Here's how the part is built. I have some questions about the finished solid (model axes, mm). Face numbers are marked on the shaded views. Round coordinates to 2 decimals unless told otherwise and drop trailing zeros. Write each loop counter-clockwise with the first axis right and the second up, starting at its lowest first coordinate (ties: lowest second). Pieces come first, ordered by that corner, then holes. Notation, with made-up numbers: (44.25, -2) - (99.25, -2) arc R22 ccw to (99.25, 35) - close; hole circle Ø8 at (67, 36). An arc over 180 degrees is marked (long way). One line per item, written item: value. Start each with the question number.
Item 1: For P1, Ø2, axis at x = 41.5, z = 2.5, coming from the -Y side; P2, Ø1, axis at x = 45, z = 2, coming from the -Y side, each with a flat end and sliding along its axis, tell me the tip position at first contact or that it passes through.
Item 2: Imagine slicing it at D-D, the plane y = -24. Please give me the cut outline in (x, z), then the cut area to 3 significant figures.
Item 3: Imagine slicing it at A-A, the plane x = 46.25. Please give me the cut outline in (y, z).
Item 4: If I drill on line 1 (X direction, y = -28, z = 0.5); line 2 (X direction, y = -22.5, z = 2.85); line 3 (X direction, y = -29.75, z = 4.3), over which ranges is the centre line in solid material (lowest first)?
Item 5: Thinking about a two-plate mould opening in X: for the marked faces 1, 2 and 3, which applies, released by +X, released by -X, zero draft, split by the parting line, or undercut?
Item 6: Imagine slicing it at B-B, the plane y = -27. Please give me the cut outline in (x, z), then the cut area to 3 significant figures.
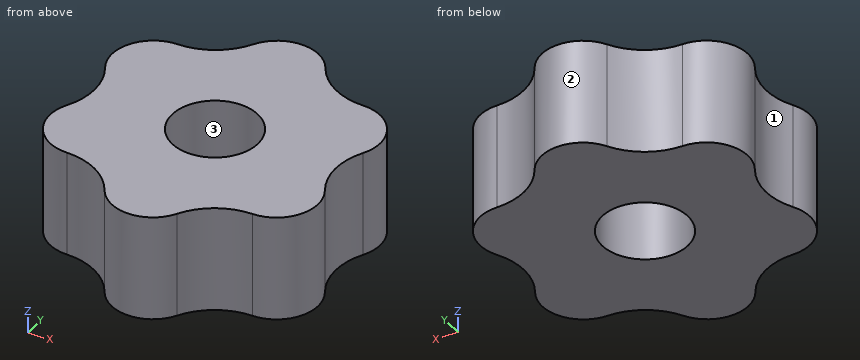
Autodesk Inventor part; units mm, degrees
ref_plane "YZ Plane" through (0, 0, 0) normal (1, 0, 0) x (0, 1, 0)
ref_plane "XZ Plane" through (0, 0, 0) normal (0, 1, 0) x (-1, 0, 0)
ref_plane "XY Plane" through (0, 0, 0) normal (0, 0, 1) x (1, 0, 0)
sketch "スケッチ1" plane through (0, 0, 0) normal (0, 0, 1) x (1, 0, 0)
  circle A0 centre (45.6488, -28.0072) radius 8
  circle A1 centre (45.6488, -28.0072) radius 7 construction
  line L0 (45.6488, -21.0072) -> (51.7109, -24.5072) construction
  line L1 (51.7109, -24.5072) -> (51.7109, -31.5072) construction
  line L2 (51.7109, -31.5072) -> (45.6488, -35.0072) construction
  line L3 (45.6488, -35.0072) -> (39.5866, -31.5072) construction
  line L4 (39.5866, -31.5072) -> (39.5866, -24.5072) construction
  line L5 (39.5866, -24.5072) -> (45.6488, -21.0072) construction
  arc A2 (47.3808, -22.0072) -> (43.9167, -22.0072) centre (45.6488, -23.0072) ccw
  arc A3 (41.3186, -23.5072) -> (39.5866, -26.5072) centre (41.3186, -25.5072) ccw
  arc A4 (39.5866, -29.5072) -> (41.3186, -32.5072) centre (41.3186, -30.5072) ccw
  arc A5 (43.9167, -34.0072) -> (47.3808, -34.0072) centre (45.6488, -33.0072) ccw
  arc A6 (49.9789, -32.5072) -> (51.7109, -29.5072) centre (49.9789, -30.5072) ccw
  arc A7 (51.7109, -26.5072) -> (49.9789, -23.5072) centre (49.9789, -25.5072) ccw
  arc A8 (47.3808, -22.0072) -> (49.9789, -23.5072) centre (49.9789, -20.5072) ccw
  arc A9 (41.3186, -23.5072) -> (43.9167, -22.0072) centre (41.3186, -20.5072) ccw
  arc A10 (39.5866, -29.5072) -> (39.5866, -26.5072) centre (36.9885, -28.0072) ccw
  arc A11 (43.9167, -34.0072) -> (41.3186, -32.5072) centre (41.3186, -35.5072) ccw
  arc A12 (49.9789, -32.5072) -> (47.3808, -34.0072) centre (49.9789, -35.5072) ccw
  arc A13 (51.7109, -26.5072) -> (51.7109, -29.5072) centre (54.309, -28.0072) ccw
  circle A14 centre (45.6488, -28.0072) radius 5.6603 construction
  circle A15 centre (45.6488, -28.0072) radius 2.025
  point P0 (0, 0)
  point P1 (51.7109, -31.5072)
  point P2 (51.7109, -24.5072)
  point P3 (51.7109, -26.5072)
  point P4 (43.9167, -22.0072)
  point P5 (41.3186, -23.5072)
  point P6 (39.5866, -26.5072)
  dimension "d5" = 14
  dimension "d4" = 16
  dimension "d6" = 360
  dimension "d7" = 360
  dimension "d8" = 11.3205
  dimension "d9" = 3
  dimension "d10" = 2
  dimension "d13" = 4.05
extrude "押し出し1" add sketch "スケッチ1" along normal blind 5 contours A8 A7 A13 A6 A12 A5 A11 A4 A10 A3 A9 A2
sketch "スケッチ2" plane through (0, 0, 5) normal (0, 0, 1) x (1, 0, 0)
  arc A0 (49.9789, -32.5072) -> (47.3808, -34.0072) centre (49.9789, -35.5072) ccw
  arc A1 (49.9789, -32.5072) -> (51.7109, -29.5072) centre (49.9789, -30.5072) ccw
  arc A2 (51.7109, -26.5072) -> (51.7109, -29.5072) centre (54.309, -28.0072) ccw
  arc A3 (51.7109, -26.5072) -> (49.9789, -23.5072) centre (49.9789, -25.5072) ccw
  arc A4 (47.3808, -22.0072) -> (49.9789, -23.5072) centre (49.9789, -20.5072) ccw
  arc A5 (47.3808, -22.0072) -> (43.9167, -22.0072) centre (45.6488, -23.0072) ccw
  arc A6 (41.3186, -23.5072) -> (43.9167, -22.0072) centre (41.3186, -20.5072) ccw
  arc A7 (41.3186, -23.5072) -> (39.5866, -26.5072) centre (41.3186, -25.5072) ccw
  arc A8 (39.5866, -29.5072) -> (39.5866, -26.5072) centre (36.9885, -28.0072) ccw
  arc A9 (39.5866, -29.5072) -> (41.3186, -32.5072) centre (41.3186, -30.5072) ccw
  arc A10 (43.9167, -34.0072) -> (41.3186, -32.5072) centre (41.3186, -35.5072) ccw
  arc A11 (43.9167, -34.0072) -> (47.3808, -34.0072) centre (45.6488, -33.0072) ccw
  circle A12 centre (45.6488, -28.0072) radius 2.025
  arc A13 (41.3186, -23.5572) -> (39.6299, -26.4822) centre (41.3186, -25.5072) ccw
  arc A14 (41.3186, -23.5572) -> (43.96, -22.0322) centre (41.3186, -20.5072) ccw
  arc A15 (47.3375, -22.0322) -> (43.96, -22.0322) centre (45.6488, -23.0072) ccw
  arc A16 (47.3375, -22.0322) -> (49.9789, -23.5572) centre (49.9789, -20.5072) ccw
  arc A17 (51.6676, -26.4822) -> (49.9789, -23.5572) centre (49.9789, -25.5072) ccw
  arc A18 (51.6676, -26.4822) -> (51.6676, -29.5322) centre (54.309, -28.0072) ccw
  arc A19 (49.9789, -32.4572) -> (51.6676, -29.5322) centre (49.9789, -30.5072) ccw
  arc A20 (49.9789, -32.4572) -> (47.3375, -33.9822) centre (49.9789, -35.5072) ccw
  arc A21 (43.96, -33.9822) -> (47.3375, -33.9822) centre (45.6488, -33.0072) ccw
  arc A22 (43.96, -33.9822) -> (41.3186, -32.4572) centre (41.3186, -35.5072) ccw
  arc A23 (39.6299, -29.5322) -> (41.3186, -32.4572) centre (41.3186, -30.5072) ccw
  arc A24 (39.6299, -29.5322) -> (39.6299, -26.4822) centre (36.9885, -28.0072) ccw
  point P0 (0, 0)
  dimension "d14" = 0.05
extrude "押し出し2" cut sketch "スケッチ2" against normal blind 10 contours A0 A11 A10 A9 A8 A7 A6 A5 A4 A3 A2 A1
properties part number "1ギア接続部" material "アルミニウム 2014-T4"
Values follow:
1. P1: stops at y = -32.7
1. P2: stops at y = -34.95
2. outline: (40.08, 0) - (51.22, 0) - (51.22, 5) - (40.08, 5) - close
2. area: 55.7 mm^2
3. outline: (-34.86, 0) - (-29.94, 0) - (-29.94, 5) - (-34.86, 5) - close; (-26.07, 0) - (-21.15, 0) - (-21.15, 5) - (-26.07, 5) - close
4. line 1: x = 40.04 to 43.62, 47.67 to 51.26
4. line 2: x = 43.63 to 47.67
4. line 3: x = 39.52 to 44.62, 46.68 to 51.78
5. face 1: released by -X
5. face 2: split by the parting line
5. face 3: undercut
6. outline: (39.87, 0) - (43.89, 0) - (43.89, 5) - (39.87, 5) - close; (47.41, 0) - (51.43, 0) - (51.43, 5) - (47.41, 5) - close
6. area: 40.2 mm^2
